```python
from build123d import *

# Parameters (mm, degrees)
SKETCH1_R           = 2.5
BOSS_EXTRUDE1_DEPTH = 100
FILLET1_R           = 1
FILLET2_R           = 0.5
FILLET3_R           = 0.5
FILLET4_R           = 0.5
FILLET5_R           = 0.5


with BuildPart() as part:
    # Sketch1 → Boss-Extrude1 (new body)
    with BuildSketch(Plane.XY):
        Polygon((13.2, 0), (13.2, 1.8), (15.45, 1.8), (15.45, 3.6), (12.95, 6.1), (7.05, 6.1), (4.55, 3.6), (4.55, 1.8), (6.8, 1.8), (6.8, 0), (0, 0), (0, 6.8), (1.8, 6.8), (1.8, 4.55), (3.6, 4.55), (6.1, 7.05), (6.1, 12.95), (3.6, 15.45), (1.8, 15.45), (1.8, 13.2), (0, 13.2), (0, 20), (6.8, 20), (6.8, 18.2), (4.55, 18.2), (4.55, 16.4), (7.05, 13.9), (12.95, 13.9), (15.45, 16.4), (15.45, 18.2), (13.2, 18.2), (13.2, 20), (20, 20), (20, 13.2), (18.2, 13.2), (18.2, 15.45), (16.4, 15.45), (13.9, 12.95), (13.9, 7.05), (16.4, 4.55), (18.2, 4.55), (18.2, 6.8), (20, 6.8), (20, 0), align=None)
        with Locations((10, 10)):
            Circle(SKETCH1_R, mode=Mode.SUBTRACT)
    extrude(amount=BOSS_EXTRUDE1_DEPTH)

    # Fillet1
    fillet1_edges = [part.edges().sort_by_distance(p)[0] for p in [
        (0, 0, 50),
        (0, 20, 50),
        (20, 20, 50),
        (20, 0, 50),
    ]]
    fillet(fillet1_edges, radius=FILLET1_R)

    # Fillet2
    fillet2_edges = [part.edges().sort_by_distance(p)[0] for p in [
        (4.55, 18.2, 50),
        (4.55, 16.4, 50),
        (7.05, 13.9, 50),
        (12.95, 13.9, 50),
        (15.45, 16.4, 50),
        (15.45, 18.2, 50),
    ]]
    fillet(fillet2_edges, radius=FILLET2_R)

    # Fillet3
    fillet3_edges = [part.edges().sort_by_distance(p)[0] for p in [
        (18.2, 15.45, 50),
        (16.4, 15.45, 50),
        (13.9, 12.95, 50),
        (13.9, 7.05, 50),
        (16.4, 4.55, 50),
        (18.2, 4.55, 50),
    ]]
    fillet(fillet3_edges, radius=FILLET3_R)

    # Fillet4
    fillet4_edges = [part.edges().sort_by_distance(p)[0] for p in [
        (1.8, 4.55, 50),
        (3.6, 4.55, 50),
        (6.1, 7.05, 50),
        (6.1, 12.95, 50),
        (3.6, 15.45, 50),
        (1.8, 15.45, 50),
    ]]
    fillet(fillet4_edges, radius=FILLET4_R)

    # Fillet5
    fillet5_edges = [part.edges().sort_by_distance(p)[0] for p in [
        (15.45, 1.8, 50),
        (15.45, 3.6, 50),
        (12.95, 6.1, 50),
        (7.05, 6.1, 50),
        (4.55, 3.6, 50),
        (4.55, 1.8, 50),
    ]]
    fillet(fillet5_edges, radius=FILLET5_R)


solid = part.part
```
Work out the finished part from the listing and answer in its coordinate system (mm). A direction names the side the tool comes from. Round coordinates to 2 decimals unless told otherwise and drop trailing zeros. Loops run counter-clockwise (first coordinate to the right, second up) from the corner with the lowest first, then second, coordinate; pieces in that order, holes last. Notation, with made-up numbers: (61, 38) -> (83, 38) arc R7 cw to (83, 51) -> close; hole circle Ø8 at (13, 76.5). An arc over 180 degrees is marked (long way). Write each question's results on one line, items separated by ' | '. Start each with the question number.
1. Section A-A (x = 10) is taken. Determine the outline of the cut face in (y, z), plus the area to 3 significant figures.
2. A tool of negligible diameter and unlimited length cuts with its end or side. For faces 3 (the face through (14, 18.2, 49)), 4 (the face through (6.8, 19, 49)), 5 (the face through (1, 6.8, 49)), 6 (the face through (20, 16, 49)), 7 (the face through (12, 12, 100)), from which of +Z, -Z, +X, -X, +Y, -Y can it reach the whole face along a straight path? Write none if from no direction.
3. For a pull along Y with two mould halves and no side action, classify faces 1 (the face through (1.8, 6, 49)), 2 (the face through (12, 12, 0)) as +Y half, -Y half, draft (parallel to the pull), parting line (faces both ways), or undercut.
4. Given pin 1 Ø10 at (x, y) = (8, 16) entering from +Z; pin 2 Ø1.5 at (y, z) = (11, 25) entering from +X; pin 3 Ø5 at (x, z) = (10, 75.5) entering from -Y; pin 4 Ø6 at (y, z) = (10, 34.5) entering from +X, each flat-ended and moving along its own axis, determine where each tip first touches the part or whether it passes through.
5. Find the intervals of material crossed by probe 1 along Y at (x, z) = (9.75, 80); probe 2 along X at (y, z) = (4.75, 93.5); probe 3 along Y at (x, z) = (17.5, 7), in increasing order. Write a range as from..to.
Evaluation:
1) outline: (6.1, 0) -> (7.5, 0) -> (7.5, 100) -> (6.1, 100) -> close; (12.5, 0) -> (13.9, 0) -> (13.9, 100) -> (12.5, 100) -> close | area: 280 mm2
2) face 3: +Z, -Z | face 4: +Z, -Z, +Y | face 5: +Z, -Z, -X | face 6: +Z, -Z, +X, +Y, -Y | face 7: +Z, +X, -X, +Y, -Y
3) face 1: undercut | face 2: draft
4) pin 1: stops at z = 100 | pin 2: stops at x = 13.9 | pin 3: stops at y = 6.1 | pin 4: stops at x = 13.97
5) probe 1: y = 6.1..7.51, 12.49..13.9 | probe 2: x = 0..1.9, 3.8..5.7, 14.3..16.2, 18.1..20 | probe 3: y = 0..4.55, 15.45..20
